Could you check a few things on this model? Use its own coordinates, in mm. Face numbers are marked on the shaded views. Coordinates: 2 decimals unless noted, no trailing zeros. Loops run counter-clockwise (first coordinate to the right, second up) from the corner with the lowest first, then second, coordinate; pieces in that order, holes last.
Autodesk Inventor part; units mm, degrees
ref_plane "YZ Plane" through (0, 0, 0) normal (1, 0, 0) x (0, 1, 0)
ref_plane "XZ Plane" through (0, 0, 0) normal (0, 1, 0) x (-1, 0, 0)
ref_plane "XY Plane" through (0, 0, 0) normal (0, 0, 1) x (1, 0, 0)
sketch "Sketch1" plane through (0, 0, 0) normal (0, 1, 0) x (-1, 0, 0)
  line L0 (45, 45) -> (-45, 45)
  line L1 (-45, 45) -> (-45, -45)
  line L2 (-45, -45) -> (45, -45)
  line L3 (45, -45) -> (45, 45)
  line L4 (45, 45) -> (-45, -45) construction
  line L5 (-45, 45) -> (45, -45) construction
  line L6 (-46, 46) -> (46, 46)
  line L7 (46, 46) -> (46, -46)
  line L8 (46, -46) -> (-46, -46)
  line L9 (-46, -46) -> (-46, 46)
  line L10 (-46, 46) -> (46, -46) construction
  line L11 (46, 46) -> (-46, -46) construction
  point P0 (0, 0)
  dimension "d0" = 90
  dimension "d1" = 90
  dimension "d2" = 92
  dimension "d3" = 92
extrude "Extrusion1" add sketch "Sketch1" along normal blind 1 contours L3 L2 L1 L0 | L6 L7 L8 L9
sketch "Sketch2" plane through (0, 1, 0) normal (0, 1, 0) x (1, 0, 0)
  line L0 (-46, -46) -> (46, -46)
  line L1 (46, -46) -> (46, 46)
  line L2 (46, 46) -> (-46, 46)
  line L3 (-46, 46) -> (-46, -46)
  line L4 (45, 45) -> (-45, 45)
  line L5 (-45, -20.5) -> (-45, -45)
  line L6 (-45, -45) -> (-17.75, -45)
  line L7 (45, -45) -> (45, 45)
  line L8 (45, 45) -> (-45, -45) construction
  line L9 (-45, 45) -> (45, -45) construction
  line L10 (-27.75, -30.5) -> (-17.75, -30.5)
  line L11 (-17.75, -30.5) -> (-17.75, -29.5)
  line L12 (-17.75, -29.5) -> (-27.75, -29.5)
  line L13 (-27.75, -29.5) -> (-27.75, -30.5)
  line L14 (-27.75, -30.5) -> (-26.75, -30.5)
  line L15 (-26.75, -30.5) -> (-26.75, -20.5)
  line L16 (-26.75, -20.5) -> (-27.75, -20.5)
  line L17 (-27.75, -20.5) -> (-27.75, -30.5)
  line L18 (-17.75, -45) -> (-17.75, -46)
  line L19 (-46, -46) -> (46, -46)
  line L20 (-45, -20.5) -> (-46, -20.5)
  point P0 (0, 0)
  dimension "d6" = 90
  dimension "d7" = 90
  dimension "d8" = 1
  dimension "d9" = 1
  dimension "d10" = 10
  dimension "d11" = 10
  dimension "d12" = 14.5
  dimension "d13" = 17.25
sketch "Sketch3" plane through (0, 1, 0) normal (0, 1, 0) x (1, 0, 0)
  line L0 (-27.75, -30.5) -> (-17.75, -30.5)
  line L1 (-27.75, -20.5) -> (-27.75, -30.5)
  line L2 (-26.75, -30.5) -> (-26.75, -20.5)
  line L3 (-17.75, -29.5) -> (-27.75, -29.5)
  line L4 (-26.75, -20.5) -> (-27.75, -20.5)
  line L5 (-17.75, -45) -> (-17.75, -46)
  line L6 (-45, -20.5) -> (-46, -20.5)
  line L7 (-46, 46) -> (-46, -46)
  line L8 (-45, -20.5) -> (-46, -20.5)
  line L9 (-46, -20.5) -> (-46, -46)
  line L10 (-46, -46) -> (-45, -46)
  line L11 (-45, -46) -> (-45, -20.5)
  line L12 (-46, -46) -> (46, -46)
  line L13 (-46, -46) -> (-17.75, -46)
  line L14 (-17.75, -46) -> (-17.75, -45)
  line L15 (-17.75, -45) -> (-46, -45)
  line L16 (-46, -45) -> (-46, -46)
  line L17 (-27.75, -30.5) -> (-17.75, -30.5)
  line L18 (-17.75, -30.5) -> (-17.75, -29.5)
  line L19 (-17.75, -29.5) -> (-27.75, -29.5)
  line L20 (-27.75, -29.5) -> (-27.75, -30.5)
  point P0 (0, 0)
extrude "Extrusion2" add sketch "Sketch3" along normal blind 7
sketch "Sketch4" plane through (-45, 1, 20.5) normal (0, 0, -1) x (-1, 0, 0)
  line L0 (-17.25, 0) -> (-18.25, 0)
  line L1 (-17.25, 0) -> (-17.25, 7)
  line L2 (-18.25, 7) -> (-17.25, 7)
  line L3 (-18.25, 0) -> (-18.25, 7)
  line L4 (1, 0) -> (0, 0)
  line L5 (1, 0) -> (1, 7)
  line L6 (0, 7) -> (1, 7)
  line L7 (0, 0) -> (0, 7)
  line L8 (0, 0) -> (-27.25, 0)
  arc A0 (-17.25, 4.027) -> (0, 4.027) centre (-8.625, 11.25) ccw
  line L9 (-91, 0) -> (1, 0)
  line L10 (-17.25, 0) -> (-17.25, 7)
  line L11 (-8.625, 0) -> (-17.25, 0)
  line L12 (-17.25, 0) -> (-17.25, 4.027)
  line L13 (0, 0) -> (0, 7)
  line L14 (-8.625, 0) -> (0, 0)
  line L15 (0, 0) -> (0, 4.027)
  point P0 (-45, -1)
  dimension "d16" = 22.5
  dimension "d17" = 8.625
extrude "Extrusion3" add sketch "Sketch4" against normal blind 10 contours A0 L7 L8 | L1 A0 L8
sketch "Sketch5" plane through (0, 1, 0) normal (0, 1, 0) x (1, 0, 0)
  line L0 (-17.75, -46) -> (46, -46)
  line L1 (-46, -20.5) -> (-46, -46)
  point P0 (0, 0)
  point P1 (-19, -19)
  dimension "d23" = 27
  dimension "d24" = 27
hole "Hole1" at (-19, 1, 19) direction (0, -1, 0) diameter 4 end through all
pattern_circular "Circular Pattern2" count 4 over 360 about axis through (0, -10, 0) along (0, 1, 0) of "Extrusion2", "Extrusion3", "Hole1"
properties part number "motor_mount_base1_template"
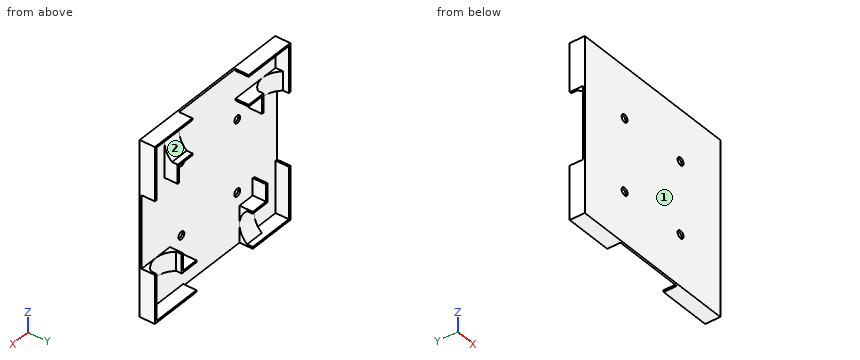
1) We'd pull the mould along X, two halves only. Please class the marked faces 1 and 2: released by +X, released by -X, zero draft, split by the parting line, or undercut.
2) Imagine slicing it at C-C on y = 6.5. State how many separate pieces and enclosed holes the cut face has, plus the area to 3 significant figures.
3) Imagine slicing it at B-B on z = 19. List the corners of the cut face in (x, y) for me, plus the area to 3 significant figures.
4) Imagine slicing it at A-A on x = -19. List the corners of the cut face in (y, z) for me.
5) If I drill on L1, parallel to X at y = 0.5, z = -19; L2, parallel to Z at x = -38, y = 1.5, over which ranges is the centre line in solid material (lowest first)?
6) Will this pin go through, and if not, where does the flat tip stop? pin 1 (5 mm diameter, centred on x = -8.5, z = 5.5, fed in from +Y).
7) Imagine slicing it at D-D on z = 32. List the corners of the cut face in (x, y) for me, plus the area to 3 significant figures.
Solved:
1. face 1: zero draft
1. face 2: undercut
2. separate pieces: 8
2. enclosed holes: 0
2. area: 287 mm2
3. outline: (-46, 0) - (-21, 0) - (-21, 1) - (-46, 1) - close; (-17, 0) - (17, 0) - (17, 1) - (-17, 1) - close; (21, 0) - (46, 0) - (46, 8) - (45, 8) - (45, 1) - (30.5, 1) - (30.5, 8) - (29.5, 8) - (29.5, 1) - (21, 1) - close
3. area: 98.0 mm2
4. outline: (0, -46) - (1, -46) - (1, -21) - (0, -21) - close; (0, -17) - (1, -17) - (1, 17) - (0, 17) - close; (0, 21) - (1, 21) - (1, 29.5) - (8, 29.5) - (8, 30.5) - (1, 30.5) - (1, 45) - (8, 45) - (8, 46) - (0, 46) - close
5. L1: x = -46 to -21, -17 to 17, 21 to 46
5. L2: z = -46 to -45, 45 to 46
6. pin 1: stops at y = 1
7. outline: (-46, 0) - (46, 0) - (46, 8) - (45, 8) - (45, 1) - (30.5, 1) - (30.5, 1.89) - (20.5, 1.89) - (20.5, 1) - (-45, 1) - (-45, 8) - (-46, 8) - close
7. area: 115 mm2
